Work out the finished part from the listing and answer in its coordinate system (mm). A direction names the side the tool comes from. Round coordinates to 2 decimals unless told otherwise and drop trailing zeros. Order: outer loops, then holes, each group sorted by start corner. A loop starts at its lowest first (then second) coordinate and runs counter-clockwise, first axis right, second up. Notation, with made-up numbers: (36.5, -22) -> (84.5, -22) arc R17 cw to (84.5, 3) -> close; hole circle Ø4 at (-21.75, 71.25). An arc over 180 degrees is marked (long way). Use a Markdown table: item, result. Add a question column.
Item 1: A cutting plane is placed at B-B, the plane x = 44.05. Give the number of separate pieces and of enclosed holes in the cut face, plus the area to 3 significant figures.
Item 2: A cutting plane is placed at C-C, the plane x = -28. Determine the outline of the cut face in (y, z), plus the area to 3 significant figures.
Item 3: A cutting plane is placed at A-A, the plane x = -8. Determine the outline of the cut face in (y, z), plus the area to 3 significant figures.
Item 4: A tool of negligible diameter and unlimited length cuts with its end or side. For faces 1 (the cylindrical face through (-47.3, -50.484, 13.028)), 2 (the flat face through (7, 42.5, 14)), 3 (the flat face through (40, 25, 4)), 4 (the flat face through (26.5, -48, 6)), 5 (the flat face through (-49.5, 32, 5)), from which of +Z, -Z, +X, -X, +Y, -Y can it reach the whole face along a straight path? Write none if from no direction.
Item 5: A cutting plane is placed at D-D, the plane y = -13. Determine the outline of the cut face in (x, z).
Item 6: For a pull along Y with two mould halves and no side action, classify faces 6 (the flat face through (-52.5, -1, 9)), 7 (the flat face through (-1, 52.5, 11)), 8 (the cylindrical face through (-44.35, 45.79, 1.97)) as +Y half, -Y half, draft (parallel to the pull), parting line (faces both ways), or undercut.
Item 7: Find the intervals of material crossed by L1, parallel to Y at x = 44.05, z = 7 (3 decimals); L2, parallel to Y at x = 44.05, z = 12.8 (3 decimals); L3, parallel to Y at x = -46.65, z = 12.6 (3 decimals), in increasing order. Write a range as [from, to].
Item 8: Flat-ended cylindrical pins translate along their axes: P1, Ø5, axis at x = -46.65, y = -47.555, coming from the +Z side; P2, Ø1.5, axis at y = 33, z = 6, coming from the +X side; P3, Ø8, axis at y = -22.5, z = 2.5, coming from the +X side; P4, Ø14, axis at x = -36.5, y = 0, coming from the -Z side. Find the tip coordinate at first contact, or state that the pin passes through.
from build123d import *

# Parameters (mm, degrees)
SKETCH_1_W           = 105
SKETCH_1_H           = 105
EXTRUDE_1_DEPTH      = 15
SKETCH_2_R           = 1.6
CUT_EXTRUDE_1_DEPTH  = 15
SKETCH_3_W           = 100
SKETCH_3_H           = 62
CUT_EXTRUDE_2_DEPTH  = 15
FILLET_1_R           = 8
SKETCH_4_OUTSIDE_W   = 136.85
SKETCH_4_OUTSIDE_H   = 136.85
SKETCH_4_OUTSIDE_R   = 2.9
CUT_EXTRUDE_3_DEPTH  = 4
SKETCH_5_W           = 51
SKETCH_5_H           = 9
CUT_EXTRUDE_4_DEPTH  = 4
SKETCH_6_W           = 57
SKETCH_6_H           = 34
CUT_EXTRUDE_5_DEPTH  = 4
CUT_EXTRUDE_6_DEPTH  = 4
FILLET_2_R           = 4
SKETCH_8_W           = 90
SKETCH_8_H           = 14
CUT_EXTRUDE_7_DEPTH  = 4
CHAMFER_1_SIZE       = 1
SKETCH_9_W           = 2
SKETCH_9_H           = 8
CUT_EXTRUDE_8_DEPTH  = 4
CHAMFER_2_SIZE       = 1
SKETCH_10_R          = 3
CUT_EXTRUDE_9_DEPTH  = 4
CUT_EXTRUDE_10_DEPTH = 5
FILLET_3_R           = 2


with BuildPart() as part:
    # 草图1 → 凸台-拉伸1 (new body)
    with BuildSketch(Plane.XY):
        Rectangle(SKETCH_1_W, SKETCH_1_H)
    extrude(amount=EXTRUDE_1_DEPTH)

    # 草图2 → 切除-拉伸1 (cut)
    with BuildSketch(Plane.XY.offset(15)):
        with Locations((-46.65, 47.555)):
            Circle(SKETCH_2_R)
        with Locations((44.05, 47.555)):
            Circle(SKETCH_2_R)
        with Locations((44.05, -47.555)):
            Circle(SKETCH_2_R)
        with Locations((-46.65, -47.555)):
            Circle(SKETCH_2_R)
    extrude(amount=-CUT_EXTRUDE_1_DEPTH, mode=Mode.SUBTRACT)

    # 草图3 → 切除-拉伸2 (cut)
    with BuildSketch(Plane.XY.offset(15)):
        with Locations((2.5, -12.5)):
            Rectangle(SKETCH_3_W, SKETCH_3_H)
    extrude(amount=-CUT_EXTRUDE_2_DEPTH, mode=Mode.SUBTRACT)

    # 圆角1
    fillet_1_edges = [part.edges().sort_by_distance(p)[0] for p in [
        (-47.5, -43.5, 7.5),
        (-47.5, 18.5, 7.5),
    ]]
    fillet(fillet_1_edges, radius=FILLET_1_R)

    # 草图4 outside → 切除-拉伸3 (cut)
    with BuildSketch(Plane(origin=(0, 0, 0), x_dir=(-1, 0, 0), z_dir=(0, 0, -1))):
        Rectangle(SKETCH_4_OUTSIDE_W, SKETCH_4_OUTSIDE_H)
        with Locations((-44.05, -47.555)):
            Circle(SKETCH_4_OUTSIDE_R, mode=Mode.SUBTRACT)
        with Locations((46.65, -47.555)):
            Circle(SKETCH_4_OUTSIDE_R, mode=Mode.SUBTRACT)
        with Locations((-44.05, 47.555)):
            Circle(SKETCH_4_OUTSIDE_R, mode=Mode.SUBTRACT)
        with Locations((46.65, 47.555)):
            Circle(SKETCH_4_OUTSIDE_R, mode=Mode.SUBTRACT)
    extrude(amount=-CUT_EXTRUDE_3_DEPTH, mode=Mode.SUBTRACT)

    # 草图5 → 切除-拉伸4 (cut)
    with BuildSketch(Plane(origin=(0, 0, 4), x_dir=(-1, 0, 0), z_dir=(0, 0, -1))):
        with Locations((-1, -48)):
            Rectangle(SKETCH_5_W, SKETCH_5_H)
    extrude(amount=-CUT_EXTRUDE_4_DEPTH, mode=Mode.SUBTRACT)

    # 草图6 → 切除-拉伸5 (cut)
    with BuildSketch(Plane(origin=(0, 0, 4), x_dir=(-1, 0, 0), z_dir=(0, 0, -1))):
        with Locations((2, 35.5)):
            Rectangle(SKETCH_6_W, SKETCH_6_H)
    extrude(amount=-CUT_EXTRUDE_5_DEPTH, mode=Mode.SUBTRACT)

    # 草图7 → 切除-拉伸6 (cut)
    with BuildSketch(Plane(origin=(0, 0, 4), x_dir=(-1, 0, 0), z_dir=(0, 0, -1))):
        Polygon((-26.5, 35.5), (-26.5, 39.5), (-52.5, 39.5), (-52.5, 31.5), (-26.5, 31.5), align=None)
    extrude(amount=-CUT_EXTRUDE_6_DEPTH, mode=Mode.SUBTRACT)

    # 圆角2
    fillet_2_edges = [part.edges().sort_by_distance(p)[0] for p in [
        (26.5, 39.5, 6),
        (26.5, 31.5, 6),
    ]]
    fillet(fillet_2_edges, radius=FILLET_2_R)

    # 草图8 → 切除-拉伸7 (cut)
    with BuildSketch(Plane.XY.offset(15)):
        with Locations((7.5, 35.5)):
            Rectangle(SKETCH_8_W, SKETCH_8_H)
    extrude(amount=-CUT_EXTRUDE_7_DEPTH, mode=Mode.SUBTRACT)

    # 倒角1
    chamfer_1_edges = [part.edges().sort_by_distance(p)[0] for p in [
        (7.5, 42.5, 11),
        (7.5, 28.5, 11),
        (-37.5, 35.5, 11),
    ]]
    chamfer(chamfer_1_edges, length=CHAMFER_1_SIZE)

    # 草图9 → 切除-拉伸8 (cut)
    with BuildSketch(Plane(origin=(0, 0, 8), x_dir=(-1, 0, 0), z_dir=(0, 0, -1))):
        with Locations((-51.5, 35.5)):
            Rectangle(SKETCH_9_W, SKETCH_9_H)
    extrude(amount=-CUT_EXTRUDE_8_DEPTH, mode=Mode.SUBTRACT)

    # 倒角2
    chamfer_2_edges = [part.edges().sort_by_distance(p)[0] for p in [
        (50.5, 35.5, 11),
        (50.5, 35.5, 8),
    ]]
    chamfer(chamfer_2_edges, length=CHAMFER_2_SIZE)

    # 草图10 → 切除-拉伸9 (cut)
    with BuildSketch(Plane.XY.offset(15)):
        with Locations((-46.65, 47.555)):
            Circle(SKETCH_10_R)
        with Locations((44.05, 47.555)):
            Circle(SKETCH_10_R)
        with Locations((44.05, -47.555)):
            Circle(SKETCH_10_R)
        with Locations((-46.65, -47.555)):
            Circle(SKETCH_10_R)
    extrude(amount=-CUT_EXTRUDE_9_DEPTH, mode=Mode.SUBTRACT)

    # 草图11 → 切除-拉伸10 (cut)
    with BuildSketch(Plane(origin=(0, 0, 4), x_dir=(-1, 0, 0), z_dir=(0, 0, -1))):
        with BuildLine():
            Line((33.5, 49.5), (41.079813737, 49.5))
            ThreePointArc((41.079813737, 49.5), (42.843240971, 43.047385809), (49.5, 42.38900542))
            Line((49.5, 42.38900542), (49.5, 21.5))
            Line((49.5, 21.5), (33.5, 21.5))
            Line((33.5, 21.5), (33.5, 49.5))
        make_face()
    extrude(amount=-CUT_EXTRUDE_10_DEPTH, mode=Mode.SUBTRACT)

    # 圆角3
    fillet_3_edges = [part.edges().sort_by_distance(p)[0] for p in [
        (-42.843240971, 43.047385809, 9),
        (-49.5, 31.94450271, 9),
        (-41.5, 21.5, 9),
        (-33.5, 35.5, 9),
        (-37.289906869, 49.5, 9),
    ]]
    fillet(fillet_3_edges, radius=FILLET_3_R)


solid = part.part
Reported:
| question | item | result |
|---|---|---|
| 1 | separate pieces | 4 |
| 1 | enclosed holes | 0 |
| 1 | area | 314 mm² |
| 2 | outline | (-52.5, 4) -> (-43.5, 4) -> (-43.5, 15) -> (-52.5, 15) -> close; (18.5, 8) -> (52.5, 8) -> (52.5, 15) -> (42.5, 15) -> (42.5, 12) -> (41.5, 11) -> (29.5, 11) -> (28.5, 12) -> (28.5, 15) -> (18.5, 15) -> close |
| 2 | area | 282 mm² |
| 3 | outline | (-52.5, 8) -> (-43.5, 8) -> (-43.5, 15) -> (-52.5, 15) -> close; (18.5, 8) -> (52.5, 8) -> (52.5, 15) -> (42.5, 15) -> (42.5, 12) -> (41.5, 11) -> (29.5, 11) -> (28.5, 12) -> (28.5, 15) -> (18.5, 15) -> close |
| 3 | area | 246 mm² |
| 4 | face 1 | +Z |
| 4 | face 2 | +Z, +X |
| 4 | face 3 | -Z, +X, -X |
| 4 | face 4 | -Z, +Y, -Y |
| 4 | face 5 | -Z |
| 5 | outline | (-52.5, 4) -> (-47.5, 4) -> (-47.5, 15) -> (-52.5, 15) -> close |
| 6 | face 6 | draft |
| 6 | face 7 | +Y half |
| 6 | face 8 | undercut |
| 7 | L1 | [-52.5, -49.155], [-45.955, -43.5], [18.5, 31.5], [39.5, 45.955], [49.155, 52.5] |
| 7 | L2 | [-52.5, -50.555], [-44.555, -43.5], [18.5, 28.5], [42.5, 44.555], [50.555, 52.5] |
| 7 | L3 | [-52.5, -50.555], [-44.555, -39.089], [14.089, 44.555], [50.555, 52.5] |
| 8 | P1 | z = 11 |
| 8 | P2 | x = -30.5 |
| 8 | P3 | x = -47.5 |
| 8 | P4 | through |
